Geometry: see drawing. Coordinates: mm, zero at the bounding-box minimum. Give positions to 0.01 mm unless a question says otherwise; leave off trailing zeros. Write each loop counter-clockwise with the first axis right and the second up, starting at its lowest first coordinate (ties: lowest second). Pieces come first, ordered by that corner, then holes. Notation, with made-up numbers: (-37.5, -23) -> (-29.5, -23) arc R17 cw to (-29.5, -5) -> close; hole circle Ø4 at (52, 65). An arc over 180 degrees is marked (long way). Use one line per item in the form item = value. Start each with the question number.
(1) Cut plane B-B, the plane y = 0.1. Output: boundary loops of the cut face in (x, z).
(2) Cut plane C-C, the plane x = 3.2. Output: boundary loops of the cut face in (y, z), and give its area (3 significant figures).
(3) First-contact query: P1, Ø2.5, axis at x = 3.2, z = 3.2, coming from the -Y side. Flat tip, straight axial feed; report the tip coordinate or a pass-through.
(4) Cut plane A-A, the plane z = 3.2. Output: boundary loops of the cut face in (x, y).
(5) Draft query along X for the marked faces 1, 2, 3 and 4. Return one class per face: pulls with the +X half, pulls with the -X half, needs draft (parallel to the pull), parting line crosses it, or undercut.
(6) Material intervals for line 1 along Z through (x, y) = (3.2, 0.5); line 2 along Z through (x, y) = (4.5, 0.1), sorted ascending. Write a range as from..to.
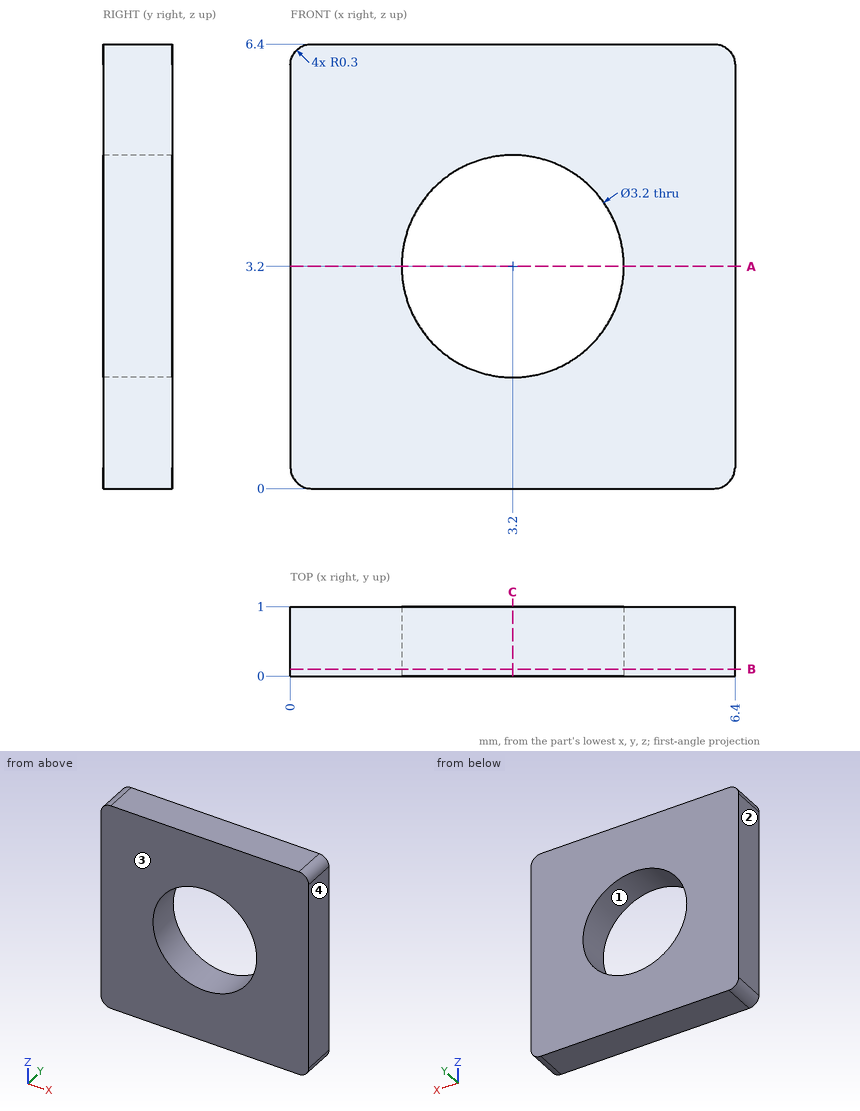
Geometry says:
q1.outline = (0, 0.3) arc R0.3 ccw to (0.3, 0) -> (6.1, 0) arc R0.3 ccw to (6.4, 0.3) -> (6.4, 6.1) arc R0.3 ccw to (6.1, 6.4) -> (0.3, 6.4) arc R0.3 ccw to (0, 6.1) -> close; hole circle Ø3.2 at (3.2, 3.2)
q2.outline = (0, 0) -> (1, 0) -> (1, 1.6) -> (0, 1.6) -> close; (0, 4.8) -> (1, 4.8) -> (1, 6.4) -> (0, 6.4) -> close
q2.area = 3.20 mm^2
q3.P1 = through
q4.outline = (0, 0) -> (1.6, 0) -> (1.6, 1) -> (0, 1) -> close; (4.8, 0) -> (6.4, 0) -> (6.4, 1) -> (4.8, 1) -> close
q5.face_1 = undercut
q5.face_2 = pulls with the -X half
q5.face_3 = needs draft
q5.face_4 = pulls with the +X half
q6.line_1 = 0..1.6, 4.8..6.4
q6.line_2 = 0..2.27, 4.13..6.4
